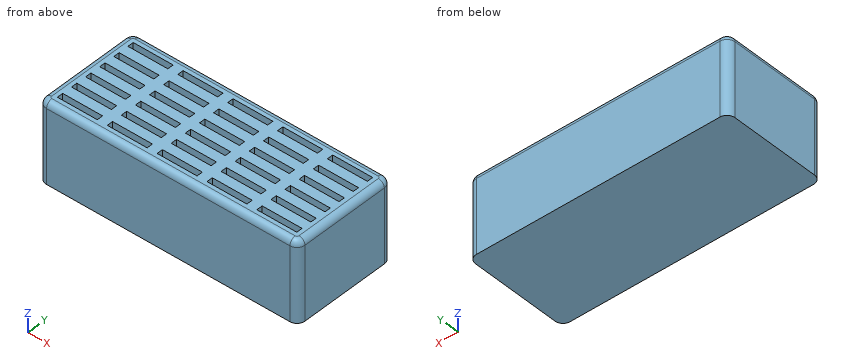
```python
from build123d import *

# Parameters (mm, degrees)
F1_DEPTH = 40
F2_W     = 20
F2_H     = 3
F3_DEPTH = 25
F4_R     = 3


with BuildPart() as f1:
    # F0 (on Top) → F1 (new body)
    with BuildSketch(Plane.XY):
        with BuildLine():
            ThreePointArc((0, 4), (1.171573, 1.171573), (4, 0))
            Line((4, 0), (126, 0))
            ThreePointArc((126, 0), (128.828427, 1.171573), (130, 4))
            Line((130, 4), (130, 49))
            ThreePointArc((130, 49), (128.828427, 51.828427), (126, 53))
            Line((126, 53), (4, 53))
            ThreePointArc((4, 53), (1.171573, 51.828427), (0, 49))
            Line((0, 49), (0, 4))
        make_face()
    extrude(amount=F1_DEPTH)

    # F2 (on face) → F3 (cut)
    with BuildSketch(Plane.XY.offset(40)):
        with Locations((15, 46.5)):
            Rectangle(F2_W, F2_H)
        with Locations((15, 38.5)):
            Rectangle(F2_W, F2_H)
        with Locations((15, 30.5)):
            Rectangle(F2_W, F2_H)
        with Locations((15, 22.5)):
            Rectangle(F2_W, F2_H)
        with Locations((15, 14.5)):
            Rectangle(F2_W, F2_H)
        with Locations((15, 6.5)):
            Rectangle(F2_W, F2_H)
        with Locations((40, 46.5)):
            Rectangle(F2_W, F2_H)
        with Locations((40, 38.5)):
            Rectangle(F2_W, F2_H)
        with Locations((40, 30.5)):
            Rectangle(F2_W, F2_H)
        with Locations((40, 22.5)):
            Rectangle(F2_W, F2_H)
        with Locations((40, 14.5)):
            Rectangle(F2_W, F2_H)
        with Locations((40, 6.5)):
            Rectangle(F2_W, F2_H)
        with Locations((65, 46.5)):
            Rectangle(F2_W, F2_H)
        with Locations((65, 38.5)):
            Rectangle(F2_W, F2_H)
        with Locations((65, 30.5)):
            Rectangle(F2_W, F2_H)
        with Locations((65, 22.5)):
            Rectangle(F2_W, F2_H)
        with Locations((65, 14.5)):
            Rectangle(F2_W, F2_H)
        with Locations((65, 6.5)):
            Rectangle(F2_W, F2_H)
        with Locations((90, 46.5)):
            Rectangle(F2_W, F2_H)
        with Locations((90, 38.5)):
            Rectangle(F2_W, F2_H)
        with Locations((90, 30.5)):
            Rectangle(F2_W, F2_H)
        with Locations((90, 22.5)):
            Rectangle(F2_W, F2_H)
        with Locations((90, 14.5)):
            Rectangle(F2_W, F2_H)
        with Locations((90, 6.5)):
            Rectangle(F2_W, F2_H)
        with Locations((115, 46.5)):
            Rectangle(F2_W, F2_H)
        with Locations((115, 38.5)):
            Rectangle(F2_W, F2_H)
        with Locations((115, 30.5)):
            Rectangle(F2_W, F2_H)
        with Locations((115, 22.5)):
            Rectangle(F2_W, F2_H)
        with Locations((115, 14.5)):
            Rectangle(F2_W, F2_H)
        with Locations((115, 6.5)):
            Rectangle(F2_W, F2_H)
    extrude(amount=-F3_DEPTH, mode=Mode.SUBTRACT)

    # F4
    f4_edges = [f1.edges().sort_by_distance(p)[0] for p in [
        (65, 53, 40),
        (1.171573, 51.828427, 40),
    ]]
    fillet(f4_edges, radius=F4_R)


solid = f1.part
```
Verification items for the finished model (mm, model axes). Give positions to 0.01 mm unless a question says otherwise; leave off trailing zeros. Answer as CSV lines item,"result". Start each with the question number.
Item 1: Gauge pin test, flat ends, axial feed: pin 1 (3.5 mm diameter, centred on x = 16, y = 6.5, fed in from +Z); pin 2 (1.5 mm diameter, centred on x = 42, y = 38.5, fed in from +Z). Record the tip position at first contact, or that the pin passes through.
Item 2: Material ranges on L1, parallel to X at y = 30, z = 29; L2, parallel to Z at x = 20.5, y = 6.5; L3, parallel to X at y = 3, z = 14, recorded low to high.
Item 3: Section check B-B, the plane z = 24. State how many separate pieces and enclosed holes the cut face has, plus the area to 3 significant figures.
Filled in:
1,pin 1,"z = 40"
1,pin 2,"z = 15"
2,L1,"0 to 5, 25 to 30, 50 to 55, 75 to 80, 100 to 105, 125 to 130"
2,L2,"0 to 15"
2,L3,"0.13 to 129.87"
3,separate pieces,"1"
3,enclosed holes,"30"
3,area,"5,080 mm^2"
